The drawing under review shows one solid part. Ordinate dimensions are in mm from its lowest x, y, z. Give positions to 0.01 mm unless a question says otherwise; leave off trailing zeros. Write each loop counter-clockwise with the first axis right and the second up, starting at its lowest first coordinate (ties: lowest second). Pieces come first, ordered by that corner, then holes. Notation, with made-up numbers: (7.25, -33) - (39.25, -33) arc R19 cw to (39.25, -5) - close; hole circle Ø10 at (0, -38.5). An arc over 180 degrees is marked (long way). Write each question's results on one line, items separated by ' | '. Start each with the question number.
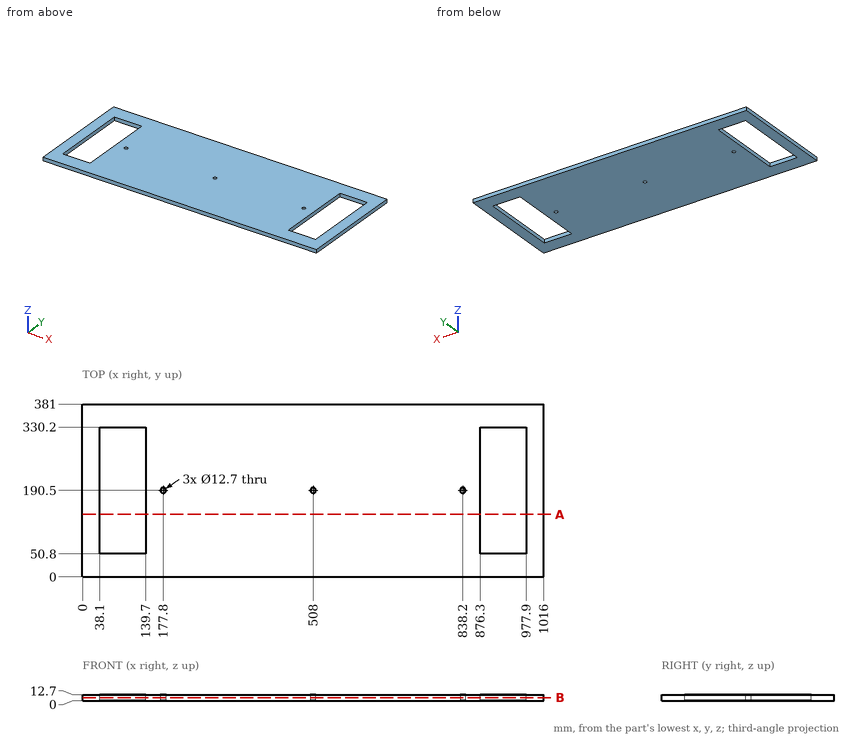
Q1. Add section B-B on z = 6.5. State the section outline as (x, y) points, plus the area to 3 significant figures.
Q2. For line 1 along X through (y, z) = (82.5, 7); line 2 along Y through (x, z) = (177.8, 9); line 3 along X through (y, z) = (193, 4), list the stretches that pass through material, from the lowest coordinate up. Write a range as [from, to].
Q3. Add section A-A on y = 138. State the section outline as (x, z) points.
Q4. Insertion check: P1, Ø10, axis at x = 508, y = 190.5, coming from the -Z side. The pin has a flat end and moves straight along its axis. Give the tip position at first contact, or say it passes through.
Result:
1) outline: (0, 0) - (1016, 0) - (1016, 381) - (0, 381) - close; hole (38.1, 50.8) - (139.7, 50.8) - (139.7, 330.2) - (38.1, 330.2) - close; hole circle Ø12.7 at (177.8, 190.5); hole circle Ø12.7 at (508, 190.5); hole circle Ø12.7 at (838.2, 190.5); hole (876.3, 50.8) - (977.9, 50.8) - (977.9, 330.2) - (876.3, 330.2) - close | area: 330,000 mm²
2) line 1: x = [0, 38.1], [139.7, 876.3], [977.9, 1016] | line 2: y = [0, 184.15], [196.85, 381] | line 3: x = [0, 38.1], [139.7, 171.96], [183.64, 502.16], [513.84, 832.36], [844.04, 876.3], [977.9, 1016]
3) outline: (0, 0) - (38.1, 0) - (38.1, 12.7) - (0, 12.7) - close; (139.7, 0) - (876.3, 0) - (876.3, 12.7) - (139.7, 12.7) - close; (977.9, 0) - (1016, 0) - (1016, 12.7) - (977.9, 12.7) - close
4) P1: passes through
